Can you work these out from the drawing? Everything is in mm from the part's minimum corner. Give positions to 0.01 mm unless a question says otherwise; leave off trailing zeros. Order: outer loops, then holes, each group sorted by start corner. A loop starts at its lowest first (then second) coordinate and runs counter-clockwise, first axis right, second up. Notation, with made-up numbers: (47, 50.25) - (101, 50.25) arc R27 cw to (101, 78.25) - close; hole circle Ø6 at (77, 5). An arc over 180 degrees is marked (long way). One line per question, with ' | ' between items.
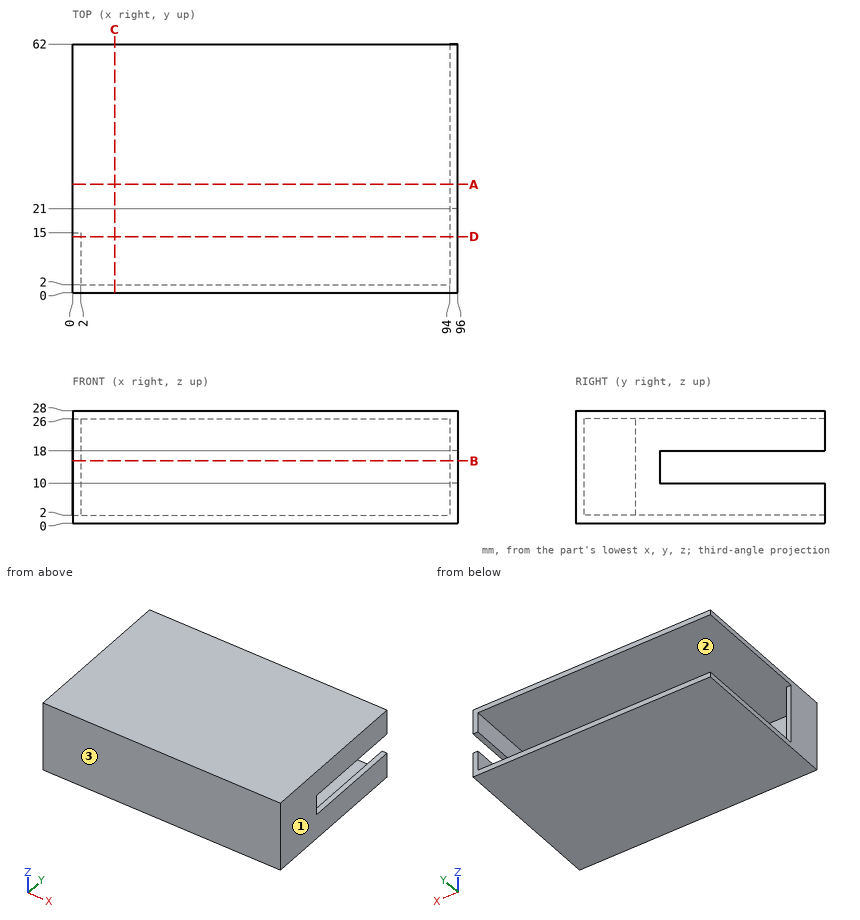
(1) Imagine slicing it at B-B (z = 15.5). List the corners of the cut face in (x, y) for me.
Answer below:
outline: (0, 0) - (96, 0) - (96, 21) - (94, 21) - (94, 2) - (2, 2) - (2, 15) - (0, 15) - close
(2) If I drill on line 1 (Z direction, x = 32.5, y = 45.5); line 2 (X direction, y = 11, z = 19.5); line 3 (X direction, y = 30, z = 24.75), over which ranges is the centre line in solid material (lowest first)?
Answer below:
line 1: 0 to 2, 26 to 28 | line 2: 0 to 2, 94 to 96 | line 3: 94 to 96
(3) Will these pins go through, and if not, where does the flat tip stop? pin 1 (7 mm diameter, centred on y = 43, z = 17, fed in from -X); pin 2 (3 mm diameter, centred on x = 43, z = 19.5, fed in from +Y); pin 3 (1 mm diameter, centred on x = 0.5, z = 15.5, fed in from +Y).
Answer below:
pin 1: x = 94 | pin 2: y = 2 | pin 3: y = 15
(4) Imagine slicing it at C-C (x = 10.5). List the corners of the cut face in (y, z) for me.
Answer below:
outline: (0, 0) - (62, 0) - (62, 2) - (2, 2) - (2, 26) - (62, 26) - (62, 28) - (0, 28) - close
(5) Imagine slicing it at A-A (y = 27). List the corners of the cut face in (x, z) for me.
Answer below:
outline: (0, 0) - (96, 0) - (96, 10) - (94, 10) - (94, 2) - (0, 2) - close; (0, 26) - (94, 26) - (94, 18) - (96, 18) - (96, 28) - (0, 28) - close
(6) Imagine slicing it at D-D (y = 14). List the corners of the cut face in (x, z) for me, and give its area (3 significant figures).
Answer below:
outline: (0, 0) - (96, 0) - (96, 28) - (0, 28) - close; hole (2, 2) - (94, 2) - (94, 26) - (2, 26) - close | area: 480 mm^2
(7) If we mould it in two halves opening along X, with no side actions, what happens to the marked faces 1, 2 and 3? For each: released by +X, released by -X, zero draft, split by the parting line, or undercut.
Answer below:
face 1: released by +X | face 2: undercut | face 3: zero draft
